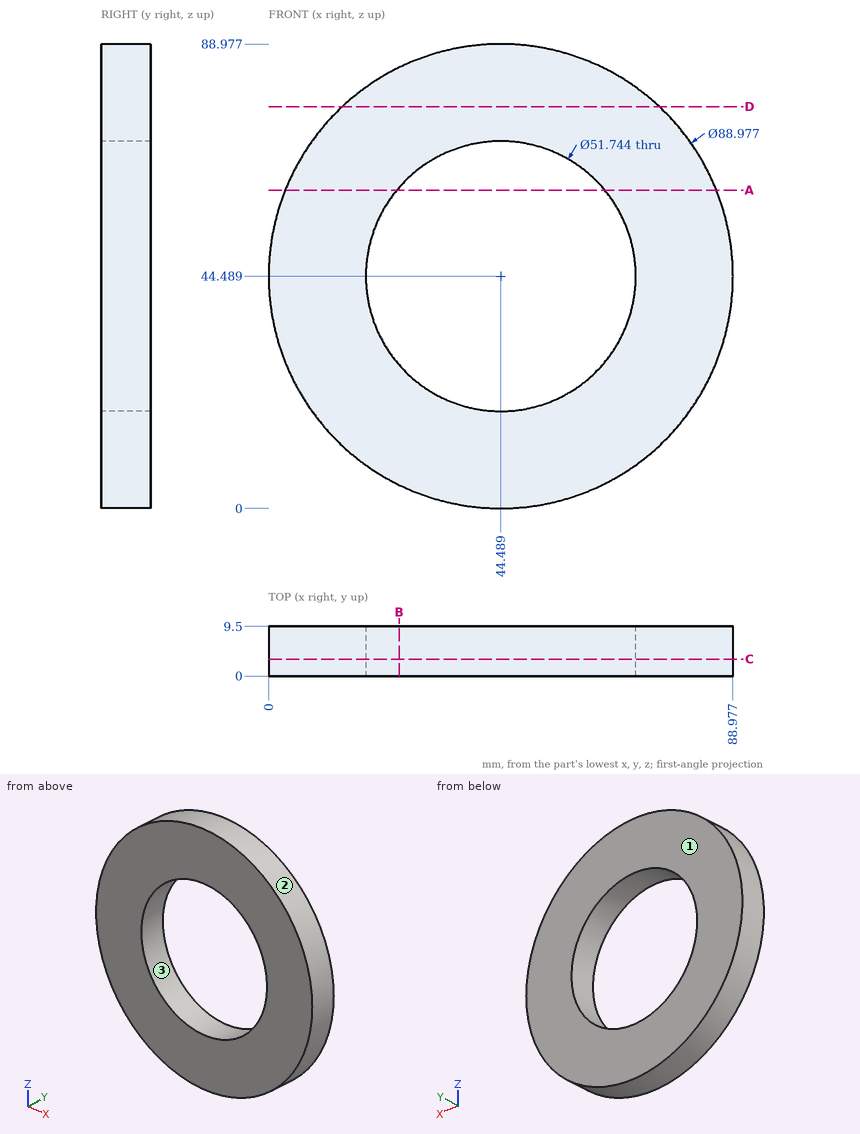
Geometry check sheet. Reference: drawing and pictorial views, mm from the part's lowest x, y, z. Coordinates: 2 decimals unless noted, no trailing zeros. Order: outer loops, then holes, each group sorted by start corner. A loop starts at its lowest first (then second) coordinate and runs counter-clockwise, first axis right, second up.
1. Sectioned sample at C-C, the plane y = 3.25. Record the cut outline in (x, z).
Results found:
outline: circle Ø88.98 at (44.49, 44.49); hole circle Ø51.74 at (44.49, 44.49)
2. Go/stop test with flat-tipped pins: pin 1 Ø1 at (x, z) = (36.5, 68.5) entering from -Y; pin 2 Ø4 at (y, z) = (8, 42) entering from +X; pin 3 Ø1 at (x, y) = (17, 1) entering from -Z; pin 4 Ø1 at (x, y) = (39, 4) entering from -Z. Record where each tip stops, or that it passes through.
Results found:
pin 1: passes through
pin 2: stops at x = 88.97
pin 3: stops at z = 9.12
pin 4: stops at z = 0.28
3. Sectioned sample at B-B, the plane x = 25. Record the cut outline in (y, z) (1 decimal).
Results found:
outline: (0, 4.5) - (9.5, 4.5) - (9.5, 27.5) - (0, 27.5) - close; (0, 61.5) - (9.5, 61.5) - (9.5, 84.5) - (0, 84.5) - close
4. Sectioned sample at D-D, the plane z = 77. Record the cut outline in (x, y), and give its area (3 significant figures).
Results found:
outline: (14.12, 0) - (74.86, 0) - (74.86, 9.5) - (14.12, 9.5) - close
area: 577 mm2
5. Sectioned sample at A-A, the plane z = 61. Record the cut outline in (x, y).
Results found:
outline: (3.18, 0) - (24.57, 0) - (24.57, 9.5) - (3.18, 9.5) - close; (64.41, 0) - (85.8, 0) - (85.8, 9.5) - (64.41, 9.5) - close
6. Release check for a two-part mould opening along X. For the marked faces 1, 2 and 3 record: +X half, -X half, draft (parallel to the pull), parting line (faces both ways), or undercut.
Results found:
face 1: draft
face 2: parting line
face 3: undercut
7. Scan lines: line 1 (Z direction, x = 45.5, y = 2) (1 decimal); line 2 (X direction, y = 2, z = 35) (1 decimal); line 3 (Z direction, x = 21.5, y = 6.25) (1 decimal). Record each from-to range of solid material in increasing order.
Results found:
line 1: z = 0 to 18.6, 70.3 to 89
line 2: x = 1 to 20.4, 68.6 to 88
line 3: z = 6.4 to 32.6, 56.4 to 82.6
